Autodesk Inventor part; units mm, degrees
ref_plane "YZ Plane" through (0, 0, 0) normal (1, 0, 0) x (0, 1, 0)
ref_plane "XZ Plane" through (0, 0, 0) normal (0, 1, 0) x (-1, 0, 0)
ref_plane "XY Plane" through (0, 0, 0) normal (0, 0, 1) x (1, 0, 0)
sketch "Sketch1" plane through (0, 0, 0) normal (0, 0, 1) x (1, 0, 0)
  circle A0 centre (0, 0) radius 10
  dimension "d0" = 20
extrude "Extrusion1" add sketch "Sketch1" along normal blind 100
sketch "Sketch2" plane through (0, 0, 100) normal (0, 0, 1) x (1, 0, 0)
  circle A0 centre (0, 0) radius 3.175
  dimension "d3" = 6.35
extrude "Extrusion2" cut sketch "Sketch2" against normal blind 20
sketch "Sketch3" plane through (0, 0, 0) normal (0, 0, -1) x (-1, 0, 0)
  circle A0 centre (0, 0) radius 3.175
  circle A1 centre (0, 0) radius 3.175
  dimension "d6" = 6.35
extrude "Extrusion3" cut sketch "Sketch3" against normal blind 20
properties part number "SupportRods"
Check sheet for the modelled part. Datum: model origin and axes. Units: mm. A direction names the side the tool comes from. Coordinates: 2 decimals unless noted, no trailing zeros. Order: outer loops, then holes, each group sorted by start corner. A loop starts at its lowest first (then second) coordinate and runs counter-clockwise, first axis right, second up. Notation, with made-up numbers: (-12, 71.5) -> (-5, 71.5) arc R38 cw to (-5, 109.5) -> close; hole circle Ø4 at (81.25, 72.25). An arc over 180 degrees is marked (long way). Write item = value, one per line. Start each with the question number.
1) Go/stop test with flat-tipped pins: P1, Ø1, axis at y = 5.5, z = 14, coming from the +X side; P2, Ø3, axis at x = 0.5, y = 0.5, coming from the +Z side; P3, Ø3, axis at y = -7, z = 27, coming from the -X side. Record where each tip stops, or that it passes through.
2) Material ranges on L1, parallel to Y at x = 0, z = 84.75 (3 decimals); L2, parallel to X at y = -2, z = 17.5; L3, parallel to X at y = 1.5, z = 88, recorded low to high.
3) Cross-section at A-A (x = 0). Enter the section's corners in (y, z) (3 decimals), then the cut area to 3 significant figures.
4) Cross-section at C-C (z = 6.5). Enter the section's corners in (x, y) (3 decimals).
5) Cross-section at D-D (z = 50). Enter the section's corners in (x, y).
6) Access from +Z, -Z, +X, -X, +Y, -Y to the whole of each face (thin tool, end or side, straight path). Record for faces 1 (the flat face through (-2.4, 2.4, 0)), 2 (the cylindrical face through (-0.69, -3.1, 90.14)), 3 (the flat face through (0, 0, 20)).
7) Mould release check, pull along X, two halves, no side actions. Record for faces 4 (the flat face through (0, 0, 80)), 5 (the cylindrical face through (0.69, -3.1, 9.86)), 6 (the flat face through (-2.4, 2.4, 100)), 7 (the cylindrical face through (-2.17, 9.76, 49.3)): +X half, -X half, draft (parallel to the pull), parting line (faces both ways), or undercut.
Ans:
q1.P1 = 8.66
q1.P2 = 80
q1.P3 = -8.35
q2.L1 = -10 to -3.175, 3.175 to 10
q2.L2 = -9.8 to -2.47, 2.47 to 9.8
q2.L3 = -9.89 to -2.8, 2.8 to 9.89
q3.outline = (-10, 0) -> (-3.175, 0) -> (-3.175, 20) -> (3.175, 20) -> (3.175, 0) -> (10, 0) -> (10, 100) -> (3.175, 100) -> (3.175, 80) -> (-3.175, 80) -> (-3.175, 100) -> (-10, 100) -> close
q3.area = 1,750 mm²
q4.outline = circle Ø20 at (0, 0); hole circle Ø6.35 at (0, 0)
q5.outline = circle Ø20 at (0, 0)
q6.face_1 = -Z, +X, -X, +Y, -Y
q6.face_2 = +Z
q6.face_3 = -Z
q7.face_4 = undercut
q7.face_5 = undercut
q7.face_6 = draft
q7.face_7 = parting line
